Autodesk Inventor part; units mm, degrees
sketch "Sketch1" plane through (0, 0, 0) normal (0, 1, 0) x (-1, 0, 0)
  line L0 (22.3723, -21.9307) -> (-45.6277, -21.9307)
  line L1 (-45.6277, -21.9307) -> (-45.6277, 74.5693)
  line L2 (-45.6277, 74.5693) -> (22.3723, 74.5693)
  line L3 (22.3723, 74.5693) -> (22.3723, -21.9307)
  point P0 (0, 0)
  dimension "d0" = 68
  dimension "d1" = 96.5
extrude "Extrusion1" add sketch "Sketch1" along normal blind 2
sketch "Sketch3" plane through (0, 2, 0) normal (0, 1, 0) x (1, 0, 0)
  line L0 (-20.3723, 21.9307) -> (43.6277, 21.9307)
  line L1 (43.6277, 21.9307) -> (43.6277, -72.5693)
  line L2 (-20.3723, -72.5693) -> (-20.3723, 21.9307)
  line L3 (45.6277, 21.9307) -> (-22.3723, 21.9307)
  line L4 (-22.3723, 21.9307) -> (-22.3723, -74.5693)
  line L5 (-22.3723, -74.5693) -> (45.6277, -74.5693)
  line L6 (45.6277, -74.5693) -> (45.6277, 21.9307)
  line L7 (-20.3723, -72.5693) -> (-20.3723, -74.5693)
  line L8 (-22.3723, -74.5693) -> (45.6277, -74.5693)
  line L9 (43.6277, -74.5693) -> (43.6277, -72.5693)
  line L10 (-18.3723, -72.5693) -> (41.6277, -72.5693)
  line L11 (41.6277, -72.5693) -> (41.6277, 21.9307)
  line L12 (41.6277, 21.9307) -> (-18.3723, 21.9307)
  line L13 (-18.3723, 21.9307) -> (-18.3723, -72.5693)
  point P0 (0, 0)
  dimension "d4" = 0
  dimension "d5" = 2
  dimension "d7" = 2
  dimension "d8" = 0
  dimension "d9" = 2
  dimension "d10" = 2
  dimension "d11" = 2
extrude "Extrusion2" add sketch "Sketch3" along normal blind 25 contours L0 L13 L10 L11 L1 L9 L5 L7 L2
sketch "Sketch4" plane through (0, 27, 0) normal (0, 1, 0) x (1, 0, 0)
  line L0 (41.6277, 21.9307) -> (41.6277, -72.5693)
  line L1 (41.6277, -72.5693) -> (-18.3723, -72.5693)
  line L2 (-18.3723, -72.5693) -> (-18.3723, 21.9307)
  line L3 (-18.3723, 21.9307) -> (-20.3723, 21.9307)
  line L4 (-20.3723, 21.9307) -> (-20.3723, -74.5693)
  line L5 (-20.3723, -74.5693) -> (43.6277, -74.5693)
  line L6 (43.6277, -74.5693) -> (43.6277, 21.9307)
  line L7 (43.6277, 21.9307) -> (41.6277, 21.9307)
  line L8 (-20.3723, 21.9307) -> (43.6277, 21.9307)
  line L9 (43.6277, 21.9307) -> (43.6277, -74.5693)
  line L10 (43.6277, -74.5693) -> (-20.3723, -74.5693)
  line L11 (-20.3723, -74.5693) -> (-20.3723, 21.9307)
  point P0 (0, 0)
extrude "Extrusion3" add sketch "Sketch4" along normal blind 2
sketch "Sketch5" plane through (0, 2, 0) normal (0, 1, 0) x (1, 0, 0)
  line L0 (43.6277, 21.9307) -> (43.6277, -74.5693)
  line L1 (43.6277, -74.5693) -> (45.6277, -74.5693)
  line L2 (45.6277, -74.5693) -> (45.6277, 21.9307)
  line L3 (45.6277, 21.9307) -> (43.6277, 21.9307)
  line L4 (-20.3723, -74.5693) -> (-20.3723, 21.9307)
  line L5 (-20.3723, 21.9307) -> (-22.3723, 21.9307)
  line L6 (-22.3723, 21.9307) -> (-22.3723, -74.5693)
  line L7 (-22.3723, -74.5693) -> (-20.3723, -74.5693)
  line L8 (-22.3723, -74.5693) -> (-20.3723, -74.5693)
  line L9 (-20.3723, -74.5693) -> (-20.3723, -72.5693)
  line L10 (-20.3723, -72.5693) -> (-22.3723, -72.5693)
  line L11 (-22.3723, -72.5693) -> (-22.3723, -74.5693)
  line L12 (43.6277, -74.5693) -> (43.6277, 21.9307)
  line L13 (45.6277, -74.5693) -> (43.6277, -74.5693)
  line L14 (43.6277, -74.5693) -> (43.6277, -72.5693)
  line L15 (43.6277, -72.5693) -> (45.6277, -72.5693)
  line L16 (45.6277, -72.5693) -> (45.6277, -74.5693)
  point P0 (0, 0)
  dimension "d16" = 2
  dimension "d17" = 2
extrude "Extrusion4" cut sketch "Sketch5" against normal blind 2 contours L15 L2 L1 L0 | L7 L6 L10 L4
sketch "Sketch6" plane through (-20.3723, 0, 74.5693) normal (-1, 0, 0) x (0, 0, 1)
  line L0 (-96.5, 29) -> (-69.5, 29)
  line L1 (-96.5, 29) -> (0, 29)
  line L2 (0, 0) -> (0, 29)
  line L3 (0, 19) -> (-59.5, 19)
  line L4 (-69.5, 29) -> (-59.5, 19)
  line L5 (-69.5, 29) -> (-55.3579, 29) construction
  line L6 (-69.5, 29) -> (0, 29)
  line L7 (0, 29) -> (0, 19)
  point P0 (-74.5693, 0)
  dimension "d20" = 27
  dimension "d21" = 10
  dimension "d22" = 45
extrude "Extrusion5" cut sketch "Sketch6" against normal up to next
sketch "Sketch7" plane through (-20.3723, 2, -21.9307) normal (-1, 0, 0) x (0, 0, 1)
  line L0 (37, 17) -> (27, 27)
  line L1 (96.5, 17) -> (37, 17)
  line L2 (29.8284, 27) -> (37.8284, 19)
  line L3 (37.8284, 19) -> (96.5, 19)
  line L4 (27, 27) -> (29.8284, 27)
  line L5 (96.5, 17) -> (96.5, 19)
  point P0 (21.9307, -2)
  dimension "d25" = 2
extrude "Extrusion6" add sketch "Sketch7" against normal up to surface (64 mm away)
sketch "Sketch13" plane through (-20.3723, 2, -21.9307) normal (-1, 0, 0) x (0, 0, 1)
  line L0 (6, 2.4048) -> (16, 2.4048)
  line L1 (16, 2.4048) -> (16, 17.4048)
  line L2 (16, 17.4048) -> (6, 17.4048)
  line L3 (6, 17.4048) -> (6, 2.4048)
  line L4 (0, 0) -> (0, 27)
  point P0 (21.9307, -2)
  dimension "d46" = 10
  dimension "d47" = 15
  dimension "d50" = 6
extrude "Extrusion7" cut sketch "Sketch13" against normal blind 2
sketch "Sketch14" plane through (0, 0, 0) normal (0, -1, 0) x (1, 0, 0)
  line L0 (-18.3723, 7.0693) -> (-18.3723, -21.9307)
  line L1 (41.6277, -21.9307) -> (41.6277, 7.0693)
  line L2 (-18.3723, -21.9307) -> (-16.3723, -21.9307)
  line L3 (-16.3723, -21.9307) -> (-16.3723, -19.9307)
  line L4 (-16.3723, -19.9307) -> (-18.3723, -19.9307)
  line L5 (-18.3723, -19.9307) -> (-18.3723, -21.9307)
  line L6 (-18.3723, -17.9307) -> (-16.3723, -17.9307)
  line L7 (-16.3723, -17.9307) -> (-16.3723, -15.9307)
  line L8 (-16.3723, -15.9307) -> (-18.3723, -15.9307)
  line L9 (-18.3723, -15.9307) -> (-18.3723, -17.9307)
  line L10 (-22.3723, -21.9307) -> (45.6277, -21.9307)
  line L11 (11.6277, -21.9307) -> (11.6277, 0)
  line L12 (39.6277, -21.9307) -> (39.6277, -19.9307)
  line L13 (39.6277, -19.9307) -> (41.6277, -19.9307)
  line L14 (41.6277, -17.9307) -> (39.6277, -17.9307)
  line L15 (39.6277, -17.9307) -> (39.6277, -15.9307)
  line L16 (39.6277, -15.9307) -> (41.6277, -15.9307)
  line L17 (39.6277, -21.9307) -> (41.6277, -21.9307)
  line L18 (41.6277, -19.9307) -> (41.6277, -21.9307)
  line L19 (41.6277, -17.9307) -> (41.6277, -15.9307)
  line L20 (41.6277, -19.9307) -> (41.6277, -17.9307)
  line L21 (39.6277, -17.9307) -> (39.6277, -19.9307)
  line L22 (-16.3723, -19.9307) -> (-16.3723, -17.9307)
  line L23 (-18.3723, -17.9307) -> (-18.3723, -19.9307)
  line L24 (-18.3723, -19.9307) -> (-16.3723, -19.9307)
  line L25 (-16.3723, -19.9307) -> (39.6277, -19.9307)
  line L26 (41.6277, 72.5693) -> (41.6277, -21.9307)
  line L27 (39.6277, -17.9307) -> (-16.3723, -17.9307)
  point P0 (0, 0)
  dimension "d51" = 2
  dimension "d52" = 2
  dimension "d53" = 2
  dimension "d54" = 2
  dimension "d55" = 2
extrude "Extrusion8" add sketch "Sketch14" against normal up to surface (27 mm away) contours L8 L7 L6 L0 | L4 L3 L2 L0 | L15 L16 L1 L14 | L13 L1 L10 L12
extrude "Extrusion10" cut sketch "Sketch14" against normal up to next contours L6 L22 L4 L0 | L27 L11 L25 L22 | L27 L21 L25 L11 | L14 L1 L13 L21
properties part number "batteri"
Verification items for the finished model (mm, model axes). A direction names the side the tool comes from. Round coordinates to 2 decimals unless told otherwise and drop trailing zeros. Loops run counter-clockwise (first coordinate to the right, second up) from the corner with the lowest first, then second, coordinate; pieces in that order, holes last. Notation, with made-up numbers: M 67,-2.75 L 110,-2.75 A18 cw 110,30.25 Z; hole C 16,-19.75 d6. An arc over 180 degrees is marked long. Write each question's results on one line, items separated by ' | '.
1) Access from +Z, -Z, +X, -X, +Y, -Y to the whole of each face (thin tool, end or side, straight path). Record for faces 5 (the flat face through (45, 2, 26)), 6 (the flat face through (-21, 2, 26)), 7 (the flat face through (-19, 19.405, -11)), 8 (the flat face through (45, 1, 72.569)), 9 (the flat face through (12, 2, -21)).
Checks:
face 5: +Z, -Z, +X, +Y | face 6: +Z, -Z, -X, +Y | face 7: -X | face 8: +Z, +X, +Y, -Y | face 9: -Z
2) Section check D-D on z = 55. Record the boundary of the cut face in (x, y), then the cut area to 3 significant figures.
Checks:
outline: M -22.37,0 L 45.63,0 L 45.63,2 L 43.63,2 L 43.63,21 L -20.37,21 L -20.37,2 L -22.37,2 Z; hole M -18.37,2 L 41.63,2 L 41.63,19 L -18.37,19 Z | area: 332 mm2
3) Section check C-C on z = 4. Record the boundary of the cut face in (x, y).
Checks:
outline: M -22.37,0 L 45.63,0 L 45.63,2 L 43.63,2 L 43.63,29 L -20.37,29 L -20.37,2 L -22.37,2 Z; hole M -18.37,2 L 41.63,2 L 41.63,27 L -18.37,27 Z
4) Section check A-A on y = 12.25. Record the boundary of the cut face in (x, z).
Checks:
outline: M -20.37,-21.93 L -16.37,-21.93 L -16.37,-19.93 L -18.37,-19.93 L -18.37,-17.93 L -16.37,-17.93 L -16.37,-15.93 L -20.37,-15.93 Z; M -20.37,-5.93 L -18.37,-5.93 L -18.37,72.57 L 41.63,72.57 L 41.63,-15.93 L 39.63,-15.93 L 39.63,-17.93 L 41.63,-17.93 L 41.63,-19.93 L 39.63,-19.93 L 39.63,-21.93 L 43.63,-21.93 L 43.63,74.57 L -20.37,74.57 Z
5) Mould release check, pull along Z, two halves, no side actions. Record for faces 1 (the flat face through (-22.372, 1, 26)), 2 (the flat face through (-21, 1, 72.569)), 3 (the flat face through (-19, 4.405, -11)), 4 (the flat face through (41.628, 13, -19)): released by +Z, released by -Z, zero draft, split by the parting line, or undercut.
Checks:
face 1: zero draft | face 2: released by +Z | face 3: undercut | face 4: undercut
6) Section check B-B on x = 21. Record the boundary of the cut face in (y, z).
Checks:
outline: M 0,-21.93 L 2,-21.93 L 2,-19.93 L 0,-19.93 Z; M 0,-17.93 L 2,-17.93 L 2,72.57 L 19,72.57 L 19,15.07 L 27,7.07 L 27,-21.93 L 29,-21.93 L 29,7.9 L 21,15.9 L 21,74.57 L 0,74.57 Z
7) Gauge pin test, flat ends, axial feed: P1, Ø3, axis at y = 10, z = -4.5, coming from the -X side; P2, Ø17.5, axis at x = -0.5, z = 34, coming from the +Y side; P3, Ø2, axis at x = 12, y = 24, coming from the +Z side. Record the tip position at first contact, or that the pin passes through.
Checks:
P1: stops at x = -20.37 | P2: stops at y = 21 | P3: stops at z = 13.9
8) Scan lines: L1, parallel to Y at x = 14, z = 34.5; L2, parallel to Y at x = 20, z = -13; L3, parallel to X at y = 16.5, z = 54. Record each from-to range of solid material in increasing order. Write a range as from..to.
Checks:
L1: y = 0..2, 19..21 | L2: y = 0..2, 27..29 | L3: x = -20.37..-18.37, 41.63..43.63
